```python
from build123d import *

# Parameters (mm, degrees)
SKETCH1_R           = 2.5
BOSS_EXTRUDE1_DEPTH = 10
BOSS_EXTRUDE2_START = -20
SKETCH2_R           = 2.5
BOSS_EXTRUDE2_DEPTH = 20


with BuildPart() as part:
    # Sketch1 → Boss-Extrude1 (new body)
    with BuildSketch(Plane(origin=(0, 0, 0), x_dir=(1, 0, 0), z_dir=(0, 1, 0))):
        Polygon((0, 15), (0, 0), (15, 0), (15, 5), (5, 5), (5, 15), align=None)
        with Locations(Location((2.879948547, 3.000793191, 0), (0, 0, 270))):
            Circle(SKETCH1_R, mode=Mode.SUBTRACT)
    extrude(amount=BOSS_EXTRUDE1_DEPTH)

    # Sketch2 → Boss-Extrude2 (add)
    with BuildSketch(Plane(origin=(0, 10, 0), x_dir=(1, 0, 0), z_dir=(0, 1, 0)).offset(BOSS_EXTRUDE2_START)):
        with Locations(Location((2.879948547, 3.000793191, 0), (0, 0, 270))):
            Circle(SKETCH2_R)
    extrude(amount=BOSS_EXTRUDE2_DEPTH)


solid = part.part
```
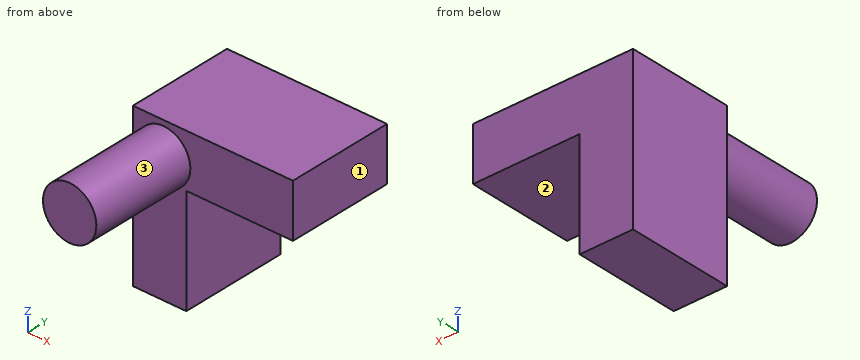
Input: part model. Units: mm. Frame: model coordinates. Face numbers are marked on the shaded views. A direction names the side the tool comes from. Round coordinates to 2 decimals unless told otherwise and drop trailing zeros. Write each loop counter-clockwise with the first axis right and the second up, starting at its lowest first coordinate (ties: lowest second). Pieces come first, ordered by that corner, then holes. Notation, with made-up numbers: M -3.75,-16.75 L 1.25,-16.75 A22 ccw 1.25,-6.75 Z; hole C 68.5,50.25 d6. An arc over 180 degrees is marked long. Write each question's results on one line, items separated by ' | '.
Q1. Section query B-B (z = -4.25). Return loops of the section in (x, y), and give its area (3 significant figures).
Results:
outline: M 0,0 L 0.71,0 L 0.71,-10 L 5.05,-10 L 5.05,0 L 15,0 L 15,10 L 0,10 Z | area: 193 mm^2
Q2. Section query C-C (y = 6.75). Return loops of the section in (x, z), and give its area (3 significant figures).
Results:
outline: M 0,-15 L 5,-15 L 5,-5 L 15,-5 L 15,0 L 0,0 Z | area: 125 mm^2
Q3. Line query: line 1 along Y through (x, z) = (8, -2.5); line 2 along X through (y, z) = (2, -10.25); line 3 along Z through (x, y) = (8.25, 4.75). Output: solid intervals per line, ascending.
Results:
line 1: y = 0 to 10 | line 2: x = 0 to 5 | line 3: z = -5 to 0
Q4. Section query D-D (z = -7.5). Return loops of the section in (x, y), and give its area (3 significant figures).
Results:
outline: M 0,0 L 5,0 L 5,10 L 0,10 Z | area: 50.0 mm^2
Q5. Pin query (flat end, axial travel): P1, Ø3, axis at x = 11.5, y = 6.5, coming from the -Z side; P2, Ø3, axis at y = -4.5, z = -8.5, coming from the -X side; P3, Ø8, axis at y = 2.5, z = -12.5, coming from the +X side. Return the tip coordinate at first contact, or that it passes through.
Results:
P1: stops at z = -5 | P2: passes through | P3: stops at x = 5
Q6. Access query for the marked faces 1, 2 and 3. Directions: +Z, -Z, +X, -X, +Y, -Y. A direction counts if a zero-diameter tool reaches every point of the face in a straight line with its end or side. Return the directions, or none.
Results:
face 1: +Z, -Z, +X, +Y, -Y | face 2: -Z, +X, +Y, -Y | face 3: -Y
Q7. Section query A-A (x = 1.5). Return loops of the section in (y, z), and give its area (3 significant figures).
Results:
outline: M -10,-5.09 L 0,-5.09 L 0,-15 L 10,-15 L 10,0 L 0,0 L 0,-0.92 L -10,-0.92 Z | area: 192 mm^2
